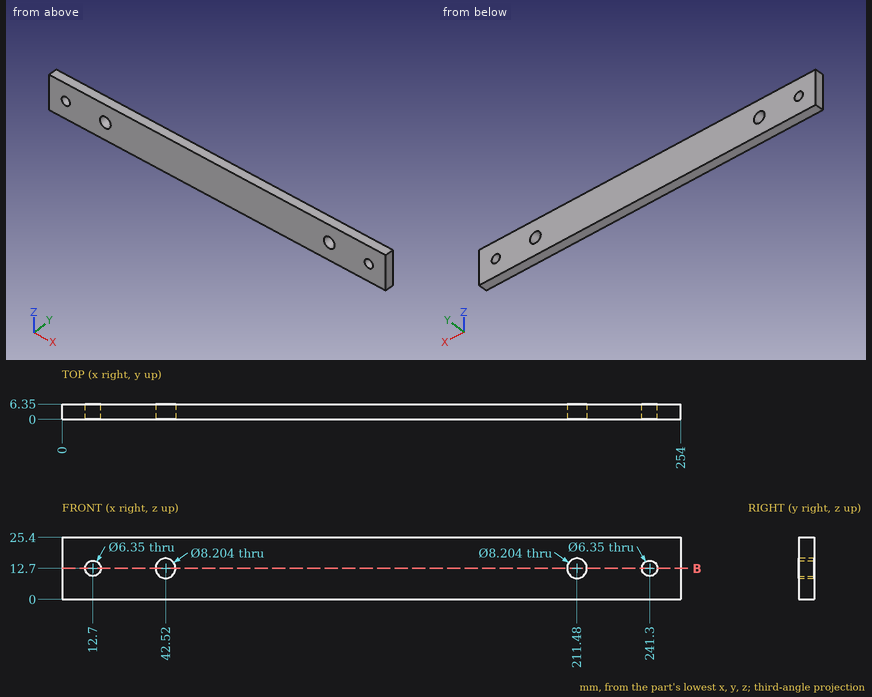
Answer from the drawing. Dimensions are ordinates in mm from the lowest x, y and z of the part. Coordinates: 2 decimals unless noted, no trailing zeros. Put each result on its own line as item: value. Start each with the question number.
Item 1: Consider probe 1 along X at (y, z) = (3.5, 12.7) (1 decimal); probe 2 along Z at (x, y) = (12.7, 3.5) (1 decimal); probe 3 along X at (y, z) = (1.75, 15.25) (1 decimal). Determine where each line is inside the solid, lowest interval first. Write a range as [from, to].
Item 2: Given pin 1 Ø5.5 at (x, z) = (12.7, 12.7) entering from -Y, flat-ended and moving along its own axis, determine where the tip first touches the part or whether it passes through.
Item 3: Section B-B, the plane z = 12.7 is taken. Count the separate pieces of the cut face and the enclosed holes in it, plus the area to 3 significant figures.
Computed:
1. probe 1: x = [0, 9.5], [15.9, 38.4], [46.6, 207.4], [215.6, 238.1], [244.5, 254]
1. probe 2: z = [0, 9.5], [15.9, 25.4]
1. probe 3: x = [0, 10.8], [14.6, 39.3], [45.7, 208.3], [214.7, 239.4], [243.2, 254]
2. pin 1: passes through
3. separate pieces: 5
3. enclosed holes: 0
3. area: 1,430 mm2
